The listing builds one solid part. Answer for the finished solid, in the listing's coordinates (mm). Face numbers are marked on the shaded views. A direction names the side the tool comes from. Give positions to 0.01 mm unless a question says otherwise; leave off trailing zeros. Write each loop counter-clockwise with the first axis right and the second up, starting at its lowest first coordinate (ties: lowest second). Pieces come first, ordered by that corner, then holes. Notation, with made-up numbers: (61.5, -24) - (69.5, -24) arc R16 cw to (69.5, -17) - close; hole circle Ø6 at (34.25, 37). An arc over 180 degrees is marked (long way). Return JSON: item names as keys, results as strings.
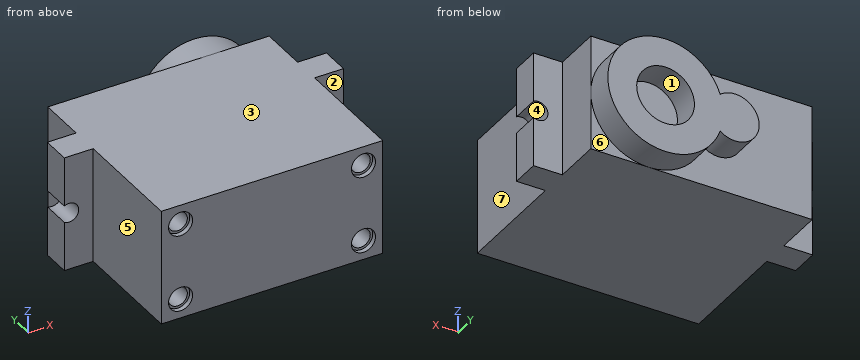
from build123d import *

# Parameters (mm, degrees)
SKETCH1_W           = 23
SKETCH1_H           = 12
SKETCH1_H_2         = 5
BOSS_EXTRUDE1_DEPTH = 6
SKETCH2_R           = 1
CUT_EXTRUDE1_DEPTH  = 22.708293346
SKETCH3_R           = 1.25
SKETCH3_R_2         = 1
CUT_EXTRUDE2_DEPTH  = 0.5
SKETCH3_2_R         = 1
CUT_EXTRUDE3_DEPTH  = 12
SKETCH4_R           = 3
BOSS_EXTRUDE2_DEPTH = 3


with BuildPart() as part:
    # Sketch1 → Boss-Extrude1 (new, symmetric)
    with BuildSketch(Plane.XY):
        with Locations((0, -6)):
            Rectangle(SKETCH1_W, SKETCH1_H)
        Polygon((-14.5, 0), (-11.5, 0), (11.5, 0), (14.5, 0), (14.5, 3), (11.5, 3), (-11.5, 3), (-14.5, 3), align=None)
        with Locations((0, 5.5)):
            Rectangle(SKETCH1_W, SKETCH1_H_2)
    extrude(amount=BOSS_EXTRUDE1_DEPTH, both=True)

    # Sketch2 → Cut-Extrude1 (cut, through all)
    with BuildSketch(Plane(origin=(0, 3, 0), x_dir=(1, 0, 0), z_dir=(0, 1, 0))):
        with Locations((14, 0)):
            Circle(SKETCH2_R)
        with Locations((-14, 0)):
            Circle(SKETCH2_R)
    extrude(amount=-CUT_EXTRUDE1_DEPTH, mode=Mode.SUBTRACT)

    # Sketch3 → Cut-Extrude2 (cut)
    # profile 1 of 4: a face of its own
    with BuildSketch(Plane.XZ.offset(12)):
        with Locations((9.5, -4)):
            Circle(SKETCH3_R)
        with Locations((9.5, -4)):
            Circle(SKETCH3_R_2, mode=Mode.SUBTRACT)
    # profile 2 of 4: a face of its own
    with BuildSketch(Plane.XZ.offset(12)):
        with Locations(Location((9.5, 4, 0), (0, 0, 180))):
            Circle(SKETCH3_R)
        with Locations(Location((9.5, 4, 0), (0, 0, 180))):
            Circle(SKETCH3_R_2, mode=Mode.SUBTRACT)
    # profile 3 of 4: a face of its own
    with BuildSketch(Plane.XZ.offset(12)):
        with Locations(Location((-9.5, -4, 0), (0, 0, 180))):
            Circle(SKETCH3_R)
        with Locations(Location((-9.5, -4, 0), (0, 0, 180))):
            Circle(SKETCH3_R_2, mode=Mode.SUBTRACT)
    # profile 4 of 4: a face of its own
    with BuildSketch(Plane.XZ.offset(12)):
        with Locations((-9.5, 4)):
            Circle(SKETCH3_R)
        with Locations((-9.5, 4)):
            Circle(SKETCH3_R_2, mode=Mode.SUBTRACT)
    extrude(amount=-CUT_EXTRUDE2_DEPTH, mode=Mode.SUBTRACT)

    # Sketch3_2 → Cut-Extrude3 (cut)
    with BuildSketch(Plane.XZ.offset(12)):
        with Locations((-9.5, -4)):
            Circle(SKETCH3_2_R)
        with Locations((-9.5, 4)):
            Circle(SKETCH3_2_R)
        with Locations((9.5, 4)):
            Circle(SKETCH3_2_R)
        with Locations((9.5, -4)):
            Circle(SKETCH3_2_R)
    extrude(amount=-CUT_EXTRUDE3_DEPTH, mode=Mode.SUBTRACT)

    # Sketch4 → Boss-Extrude2 (add)
    with BuildSketch(Plane(origin=(0, 8, 0), x_dir=(1, 0, 0), z_dir=(0, 1, 0))):
        with BuildLine():
            ThreePointArc((-0.171650012, -1.957648115), (11.5, 0), (-0.171650012, 1.957648115))
            ThreePointArc((-0.171650012, 1.957648115), (-4.226517806, 0), (-0.171650012, -1.957648115))
        make_face()
        with Locations(Location((5.5, 0, 0), (0, 0, 270))):
            Circle(SKETCH4_R, mode=Mode.SUBTRACT)
    extrude(amount=BOSS_EXTRUDE2_DEPTH)


solid = part.part
Item 1: Flat-ended cylindrical pins translate along their axes: P1, Ø5.5, axis at x = 5.5, z = 0, coming from the +Y side; P2, Ø2, axis at y = -9.5, z = -4.5, coming from the -X side; P3, Ø6, axis at x = 6, z = 0, coming from the +Y side; P4, Ø1.5, axis at x = 13.5, z = 0, coming from the -Y side. Find the tip coordinate at first contact, or state that the pin passes through.
Answer below:
{"P1": "stops at y = 8", "P2": "stops at x = -11.5", "P3": "stops at y = 11", "P4": "stops at y = 0"}
Item 2: A cutting plane is placed at C-C on z = -1.5. Determine the outline of the cut face in (x, y), then the cut area to 3 significant figures.
Answer below:
{"outline": "(-14.5, 0) - (-11.5, 0) - (-11.5, -12) - (11.5, -12) - (11.5, 0) - (14.5, 0) - (14.5, 3) - (11.5, 3) - (11.5, 8) - (11.31, 8) - (11.31, 11) - (8.1, 11) - (8.1, 8) - (2.9, 8) - (2.9, 11) - (-3.73, 11) - (-3.73, 8) - (-11.5, 8) - (-11.5, 3) - (-14.5, 3) - close", "area": "508 mm²"}
Item 3: A cutting plane is placed at A-A on y = -1.5. Determine the outline of the cut face in (x, z), then the cut area to 3 significant figures.
Answer below:
{"outline": "(-11.5, -6) - (11.5, -6) - (11.5, 6) - (-11.5, 6) - close; hole circle Ø2 at (-9.5, -4); hole circle Ø2 at (-9.5, 4); hole circle Ø2 at (9.5, -4); hole circle Ø2 at (9.5, 4)", "area": "263 mm²"}
Item 4: A cutting plane is placed at D-D on x = -9.5. Determine the outline of the cut face in (y, z).
Answer below:
{"outline": "(-12, -6) - (8, -6) - (8, 6) - (-12, 6) - (-12, 5.25) - (-11.5, 5.25) - (-11.5, 5) - (0, 5) - (0, 3) - (-11.5, 3) - (-11.5, 2.75) - (-12, 2.75) - (-12, -2.75) - (-11.5, -2.75) - (-11.5, -3) - (0, -3) - (0, -5) - (-11.5, -5) - (-11.5, -5.25) - (-12, -5.25) - close"}
Item 5: Consider L1, parallel to Z at x = -9.5, y = -5.5; L2, parallel to X at y = -6.75, z = 4.5; L3, parallel to Y at x = -9, z = 5.75. Determine where each line is inside the solid, lowest interval first.
Answer below:
{"L1": "z = -6 to -5, -3 to 3, 5 to 6", "L2": "x = -11.5 to -10.37, -8.63 to 8.63, 10.37 to 11.5", "L3": "y = -12 to 8"}
Item 6: For the marked faces 5, 6 and 7, determine the directions among +Z, -Z, +X, -X, +Y, -Y from which every point of the face is accessible in a straight line to the end or side of a thin tool.
Answer below:
{"face 5": "+Z, -Z, -X, -Y", "face 6": "-Z, +X, +Y", "face 7": "+Z, -Z, +X, -Y"}
Item 7: The mould has two halves that part along Z. Classify the marked faces 1, 2, 3 and 4: +Z half, -Z half, draft (parallel to the pull), parting line (faces both ways), or undercut.
Answer below:
{"face 1": "undercut", "face 2": "draft", "face 3": "+Z half", "face 4": "undercut"}
Item 8: A cutting plane is placed at B-B on x = -14. Determine the outline of the cut face in (y, z), then the cut area to 3 significant figures.
Answer below:
{"outline": "(0, -6) - (3, -6) - (3, -1) - (0, -1) - close; (0, 1) - (3, 1) - (3, 6) - (0, 6) - close", "area": "30.0 mm²"}
